Read the model definition and answer for the solid it produces. Units are mm, in the model's axes. A direction names the side the tool comes from. Coordinates: 2 decimals unless noted, no trailing zeros. Write each loop counter-clockwise with the first axis right and the second up, starting at its lowest first coordinate (ties: lowest second). Pieces come first, ordered by that corner, then holes. Notation, with made-up numbers: (41, 23.5) - (55, 23.5) arc R10 cw to (55, 39.5) - close; hole circle Ø3 at (-22, 13). An arc over 180 degrees is marked (long way). Return JSON: item names as keys, results as strings.
```python
from build123d import *

# Parameters (mm, degrees)
BOSS_EXTRUDE1_DEPTH = 76.2
CUT_EXTRUDE1_START  = -3.175
SKETCH2_R           = 3.175
SKETCH2_R_2         = 2.921
CUT_EXTRUDE1_DEPTH  = 0.7874
CUT_EXTRUDE2_START  = -6.35
SKETCH3_R           = 3.175
SKETCH3_R_2         = 2.921
CUT_EXTRUDE2_DEPTH  = 0.7874
CUT_EXTRUDE3_START  = -23.04415
SKETCH3_5_R         = 3.175
SKETCH3_5_R_2       = 2.921
CUT_EXTRUDE3_DEPTH  = 0.7874
CUT_EXTRUDE4_START  = -28.575
SKETCH3_6_R         = 3.175
SKETCH3_6_R_2       = 2.921
CUT_EXTRUDE4_DEPTH  = 0.7874


with BuildPart() as part:
    # Sketch1 → Boss-Extrude1 (new body)
    with BuildSketch(Plane(origin=(0, 0, 0), x_dir=(1, 0, 0), z_dir=(0, 1, 0))):
        with BuildLine():
            Line((-1.190625, 2.943303775), (-1.190625, 1.752678775))
            Line((-1.190625, 1.752678775), (1.190625, 1.752678775))
            Line((1.190625, 1.752678775), (1.190625, 2.943303775))
            ThreePointArc((1.190625, 2.943303775), (0, -3.175), (-1.190625, 2.943303775))
        make_face()
    extrude(amount=BOSS_EXTRUDE1_DEPTH)

    # Sketch2 → Cut-Extrude1 (cut)
    with BuildSketch(Plane(origin=(0, 76.2, 0), x_dir=(1, 0, 0), z_dir=(0, 1, 0)).offset(CUT_EXTRUDE1_START)):
        Circle(SKETCH2_R)
        Circle(SKETCH2_R_2, mode=Mode.SUBTRACT)
    extrude(amount=CUT_EXTRUDE1_DEPTH, mode=Mode.SUBTRACT)

    # Sketch3 → Cut-Extrude2 (cut)
    with BuildSketch(Plane.XZ.offset(CUT_EXTRUDE2_START)):
        Circle(SKETCH3_R)
        Circle(SKETCH3_R_2, mode=Mode.SUBTRACT)
    extrude(amount=CUT_EXTRUDE2_DEPTH, mode=Mode.SUBTRACT)

    # Sketch3<5> → Cut-Extrude3 (cut)
    with BuildSketch(Plane.XZ.offset(CUT_EXTRUDE3_START)):
        Circle(SKETCH3_5_R)
        Circle(SKETCH3_5_R_2, mode=Mode.SUBTRACT)
    extrude(amount=CUT_EXTRUDE3_DEPTH, mode=Mode.SUBTRACT)

    # Sketch3<6> → Cut-Extrude4 (cut)
    with BuildSketch(Plane.XZ.offset(CUT_EXTRUDE4_START)):
        Circle(SKETCH3_6_R)
        Circle(SKETCH3_6_R_2, mode=Mode.SUBTRACT)
    extrude(amount=CUT_EXTRUDE4_DEPTH, mode=Mode.SUBTRACT)


solid = part.part
```
(1) Determine the mould class of faces 4 (the face through (0, 76.2, 0)), 5 (the face through (-0.11, 73.41, 2.92)), 6 (the face through (-1.191, 38, -2)), 7 (the face through (0.11, 28.19, 2.92)) for opening direction Y: +Y half, -Y half, draft (parallel to the pull), parting line (faces both ways), or undercut.
Answer:
{"face 4": "+Y half", "face 5": "undercut", "face 6": "draft", "face 7": "undercut"}
(2) A cutting plane is placed at A-A (x = 0). Determine the outline of the cut face in (y, z) (3 decimals).
Answer:
{"outline": "(0, -1.753) - (76.2, -1.753) - (76.2, 3.175) - (73.812, 3.175) - (73.812, 2.921) - (73.025, 2.921) - (73.025, 3.175) - (28.575, 3.175) - (28.575, 2.921) - (27.788, 2.921) - (27.788, 3.175) - (23.044, 3.175) - (23.044, 2.921) - (22.257, 2.921) - (22.257, 3.175) - (6.35, 3.175) - (6.35, 2.921) - (5.563, 2.921) - (5.563, 3.175) - (0, 3.175) - close"}
(3) Flat-ended cylindrical pins translate along their axes: P1, Ø1.2, axis at x = 0.5, y = 41, coming from the -Z side; P2, Ø1, axis at x = 2, y = 8.5, coming from the -Z side; P3, Ø1.3, axis at y = 45.5, z = -2.5, coming from the -X side. Find the tip coordinate at first contact, or state that the pin passes through.
Answer:
{"P1": "z = -1.75", "P2": "z = -2.8", "P3": "x = -2.58"}
(4) Straight lines are drawn through the part: line 1 (X direction, y = 23.5, z = 1.25); line 2 (Z direction, x = 0, y = 19) (3 decimals); line 3 (X direction, y = 8.5, z = -2). For each, find the intervals that lie inside material, in ascending order. Write a range as from..to.
Answer:
{"line 1": "-2.92..2.92", "line 2": "-1.753..3.175", "line 3": "-2.47..-1.19, 1.19..2.47"}
(5) Which of the six approach directions +Z, -Z, +X, -X, +Y, -Y give full straight-line access (tool end or side, diameter ignored) to faces 1 (the face through (0.123, 25.383, 3.173)), 2 (the face through (0.11, 5.96, 2.92)), 3 (the face through (1.191, 38, -2))?
Answer:
{"face 1": "+Y, -Y", "face 2": "none", "face 3": "-Z, +Y, -Y"}
(6) A cutting plane is placed at B-B (y = 34.5). Determine the outline of the cut face in (x, z) (3 decimals), and give its area (3 significant figures).
Answer:
{"outline": "(-1.191, -2.943) - (-1.191, -1.753) - (1.191, -1.753) - (1.191, -2.943) arc R3.175 ccw (long way) to start", "area": "28.5 mm²"}
